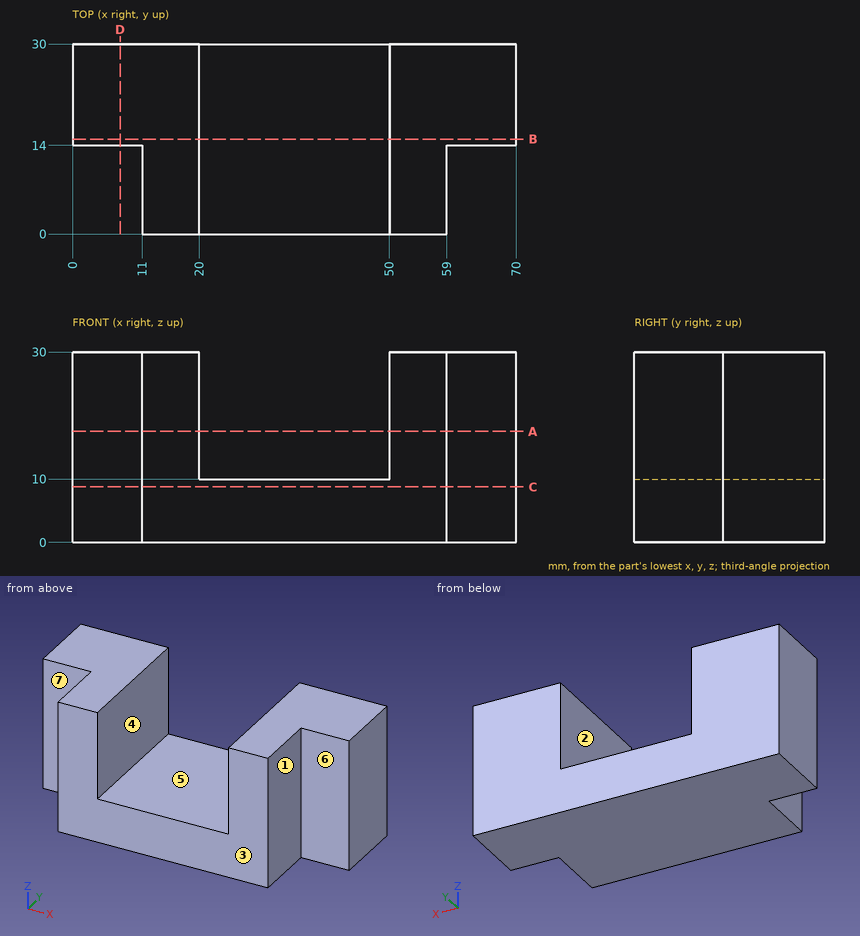
Check sheet for the drawn part. Datum: minimum x, y, z corner. Units: mm. A direction names the side the tool comes from. Round coordinates to 2 decimals unless told otherwise and drop trailing zeros. Write each loop counter-clockwise with the first axis right and the second up, starting at its lowest first coordinate (ties: lowest second). Pieces come first, ordered by that corner, then holes. Notation, with made-up numbers: (60.25, 51.25) -> (115.25, 51.25) arc R8 ccw to (115.25, 58.25) -> close; hole circle Ø1 at (55, -36.75). An arc over 180 degrees is marked (long way). Write each question's results on one line, items separated by ' | '. Start each with the question number.
1. Cross-section at A-A (z = 17.5). Enter the section's corners in (x, y), then the cut area to 3 significant figures.
2. Cross-section at B-B (y = 15). Enter the section's corners in (x, z).
3. Depth check by flat-ended pin: P1, Ø2, axis at x = 48.5, y = 15, coming from the +Z side; P2, Ø5.5, axis at x = 67, z = 12.5, coming from the -Y side; P3, Ø7, axis at y = 4.5, z = 9.5, coming from the -X side. Enter the tip coordinate at first touch or a pass-through.
4. Set-up check for the marked faces 5, 6 and 7: record each of +Z, -Z, +X, -X, +Y, -Y from which the full face is reachable in a straight line by a thin tool's end or side.
5. Material ranges on probe 1 along X at (y, z) = (22, 27.5); probe 2 along X at (y, z) = (12.5, 16.75); probe 3 along Z at (x, y) = (39.5, 25), recorded low to high. Write a range as from..to.
6. Cross-section at D-D (x = 7.5). Enter the section's corners in (y, z), then the cut area to 3 significant figures.
7. Cross-section at C-C (z = 8.75). Enter the section's corners in (x, y).
8. Draft check along X on the marked faces 1, 2, 3 and 4. Enter one of: +X half, -X half, draft (parallel to the pull), parting line (faces both ways), or undercut.
Solutions:
1) outline: (0, 14) -> (11, 14) -> (11, 0) -> (20, 0) -> (20, 30) -> (0, 30) -> close; (50, 0) -> (59, 0) -> (59, 14) -> (70, 14) -> (70, 30) -> (50, 30) -> close | area: 892 mm2
2) outline: (0, 0) -> (70, 0) -> (70, 30) -> (50, 30) -> (50, 10) -> (20, 10) -> (20, 30) -> (0, 30) -> close
3) P1: stops at z = 10 | P2: stops at y = 14 | P3: stops at x = 11
4) face 5: +Z, +Y, -Y | face 6: +Z, -Z, +X, -Y | face 7: +Z, -Z, -X, -Y
5) probe 1: x = 0..20, 50..70 | probe 2: x = 11..20, 50..59 | probe 3: z = 0..10
6) outline: (14, 0) -> (30, 0) -> (30, 30) -> (14, 30) -> close | area: 480 mm2
7) outline: (0, 14) -> (11, 14) -> (11, 0) -> (59, 0) -> (59, 14) -> (70, 14) -> (70, 30) -> (0, 30) -> close
8) face 1: +X half | face 2: undercut | face 3: draft | face 4: undercut
